```python
from build123d import *

# Parameters (mm, degrees)
EXTRUDE_1_DEPTH     = 105
SKETCH_23_W         = 30
SKETCH_23_H         = 10
CUT_EXTRUDE_1_DEPTH = 25
SKETCH_24_R         = 42.5
CUT_EXTRUDE_3_DEPTH = 35


with BuildPart() as part:
    # Эскиз2 → Бобышка-Вытянуть1 (new body)
    with BuildSketch(Plane(origin=(0, 0, 0), x_dir=(0, 0, -1), z_dir=(1, 0, 0))):
        Polygon((0, 0), (0, -85), (-80, -85), (-80, -50), (-20, -50), (-20, -25), (-30, -25), (-30, 0), align=None)
    extrude(amount=EXTRUDE_1_DEPTH)

    # Эскиз23 → Вырез-Вытянуть1 (cut)
    with BuildSketch(Plane(origin=(0, 0, 0), x_dir=(1, 0, 0), z_dir=(0, 1, 0))):
        with Locations((52.5, -25)):
            Rectangle(SKETCH_23_W, SKETCH_23_H)
    extrude(amount=-CUT_EXTRUDE_1_DEPTH, mode=Mode.SUBTRACT)

    # Эскиз24 → Вырез-Вытянуть3 (cut)
    with BuildSketch(Plane(origin=(0, -50, 0), x_dir=(1, 0, 0), z_dir=(0, 1, 0))):
        with Locations((52.5, -80)):
            Circle(SKETCH_24_R)
    extrude(amount=-CUT_EXTRUDE_3_DEPTH, mode=Mode.SUBTRACT)


solid = part.part
```
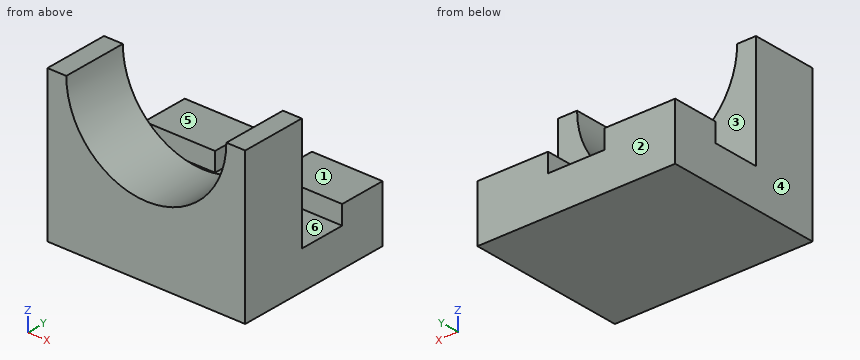
For this review, take the finished solid that the model builds, in its own axes (mm). Face numbers are marked on the shaded views. A direction names the side the tool comes from. Round coordinates to 2 decimals unless told otherwise and drop trailing zeros. Write each loop counter-clockwise with the first axis right and the second up, starting at its lowest first coordinate (ties: lowest second). Pieces come first, ordered by that corner, then holes. Notation, with made-up numbers: (-23.75, 51.5) - (29.25, 51.5) arc R15 cw to (29.25, 55.5) - close; hole circle Ø10 at (-20, -19.75). An arc over 180 degrees is marked (long way). Answer as CSV lines item,"result". Start each with the question number.
(1) Add section D-D, the plane z = 59. State the section outline as (x, y) points.
(2) Add section A-A, the plane z = 22. State the section outline as (x, y) points, plus the area to 3 significant figures.
(3) For pin 1 (3 mm diameter, centred on y = -15.5, z = 23.5, fed in from -X); pin 2 (6 mm diameter, centred on x = 23.5, y = -13.5, fed in from +Z); pin 3 (12 mm diameter, centred on y = -12, z = 37.5, fed in from +X); pin 4 (3 mm diameter, centred on x = 29.5, z = 42, fed in from +Y), all flat-tipped, find the tip position at first contact; note any pin that passes through.
(4) Add section C-C, the plane x = 34. State the section outline as (y, z) points.
(5) Machinability: for the marked faces 1, 2 and 3, which of the approach directions +Z, -Z, +X, -X, +Y, -Y give a long, thin tool a straight path to every point of the face, cutting with its end or side? Answer none if there is none.
(6) Add section B-B, the plane y = -10. State the section outline as (x, z) points, plus the area to 3 significant figures.
(7) Mouldability with a two-part tool opening along X and no side actions: class the marked faces 4, 5 and 6 as +X half, -X half, draft (parallel to the pull), parting line (faces both ways), or undercut.
(8) For line 1 (Z direction, x = 88, y = -19); line 2 (Z direction, x = 41.5, y = -43); line 3 (X direction, y = -80.5, z = 72), list the stretches that pass through material, from the lowest coordinate up.
From the geometry:
1,outline,"(0, -85) - (15.55, -85) - (15.55, -50) - (0, -50) - close; (89.45, -85) - (105, -85) - (105, -50) - (89.45, -50) - close"
2,outline,"(0, -85) - (105, -85) - (105, -50) - (0, -50) - close; (0, -25) - (37.5, -25) - (37.5, 0) - (0, 0) - close; (67.5, -25) - (105, -25) - (105, 0) - (67.5, 0) - close"
2,area,"5,550 mm²"
3,pin 1,"stops at x = 0"
3,pin 2,"stops at z = 30"
3,pin 3,"passes through"
3,pin 4,"stops at y = -50"
4,outline,"(-85, 0) - (0, 0) - (0, 30) - (-25, 30) - (-25, 20) - (-50, 20) - (-50, 41.74) - (-85, 41.74) - close"
5,face 1,"+Z, +X, -X, +Y"
5,face 2,"+Z, -Z, +X, -X, +Y"
5,face 3,"+Z, +X, -X"
6,outline,"(0, 0) - (105, 0) - (105, 30) - (67.5, 30) - (67.5, 20) - (37.5, 20) - (37.5, 30) - (0, 30) - close"
6,area,"2,850 mm²"
7,face 4,"-X half"
7,face 5,"draft"
7,face 6,"undercut"
8,line 1,"z = 0 to 30"
8,line 2,"z = 0 to 20"
8,line 3,"x = 0 to 10.76, 94.24 to 105"
